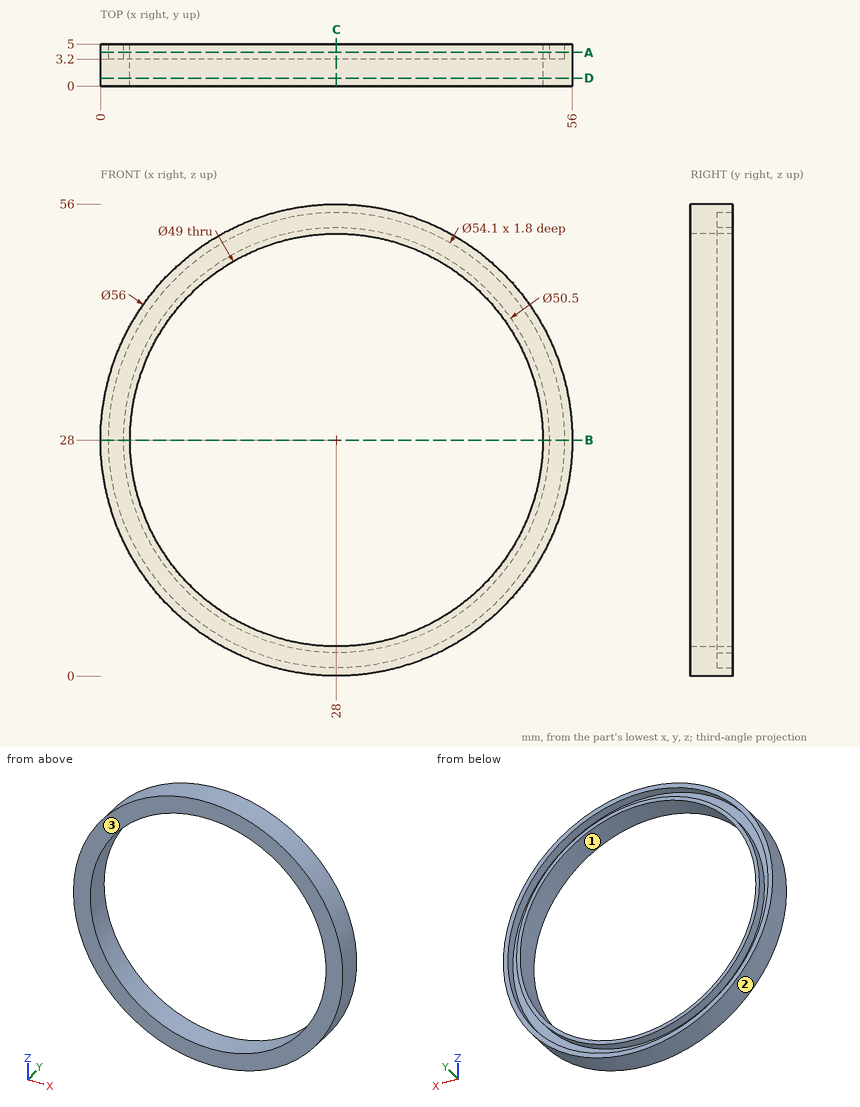
Input: dimensioned drawing with shaded views. Units: mm. Origin: part minimum x, y, z. Coordinates: 2 decimals unless noted, no trailing zeros. Order: outer loops, then holes, each group sorted by start corner. A loop starts at its lowest first (then second) coordinate and runs counter-clockwise, first axis right, second up.
(1) Section query A-A (y = 4). Return the cut outline in (x, z), plus the area to 3 significant figures.
(2) Section query C-C (x = 28). Return the cut outline in (y, z).
(3) Section query D-D (y = 0.95). Return the cut outline in (x, z), plus the area to 3 significant figures.
(4) First-contact query: pin 1 (1.5 mm diameter, centred on x = 24, y = 1.5, fed in from -Z); pin 2 (2 mm diameter, centred on x = 31, y = 4.5, fed in from -Z). Flat tips, straight axial feed; report the tip coordinate or a pass-through.
(5) Material intervals for probe 1 along Z at (x, y) = (28, 4.65); probe 2 along Z at (x, y) = (13.5, 3.9); probe 3 along X at (y, z) = (3.5, 19), sorted ascending.
(6) Section query B-B (z = 28). Return the cut outline in (x, y).
(7) Draft query along Z for the marked faces 1, 2 and 3. Return one class per face: pulls with the +Z half, pulls with the -Z half, needs draft (parallel to the pull), parting line crosses it, or undercut.
Solution:
1. outline: circle Ø56 at (28, 28); circle Ø50.5 at (28, 28); hole circle Ø54.1 at (28, 28); hole circle Ø49 at (28, 28)
1. area: 282 mm2
2. outline: (0, 0) - (5, 0) - (5, 0.95) - (3.2, 0.95) - (3.2, 2.75) - (5, 2.75) - (5, 3.5) - (0, 3.5) - close; (0, 52.5) - (5, 52.5) - (5, 53.25) - (3.2, 53.25) - (3.2, 55.05) - (5, 55.05) - (5, 56) - (0, 56) - close
3. outline: circle Ø56 at (28, 28); hole circle Ø49 at (28, 28)
3. area: 577 mm2
4. pin 1: stops at z = 0.19
4. pin 2: stops at z = 0.07
5. probe 1: z = 0 to 0.95, 2.75 to 3.5, 52.5 to 53.25, 55.05 to 56
5. probe 2: z = 4.05 to 5.16, 7.33 to 8.25, 47.75 to 48.67, 50.84 to 51.95
5. probe 3: x = 1.49 to 2.49, 4.41 to 5.21, 50.79 to 51.59, 53.51 to 54.51
6. outline: (0, 0) - (3.5, 0) - (3.5, 5) - (2.75, 5) - (2.75, 3.2) - (0.95, 3.2) - (0.95, 5) - (0, 5) - close; (52.5, 0) - (56, 0) - (56, 5) - (55.05, 5) - (55.05, 3.2) - (53.25, 3.2) - (53.25, 5) - (52.5, 5) - close
7. face 1: undercut
7. face 2: parting line crosses it
7. face 3: needs draft
